from build123d import *

# Parameters (mm, degrees)
F1_DEPTH = 3.75
F2_R     = 1.25
F3_DEPTH = 30


with BuildPart() as f1:
    # F0 (on Front) → F1 (new body)
    with BuildSketch(Plane.XZ):
        Polygon((6.409004, 25.153901), (-3.681577, 25.153901), (-7.50148, 17.153901), (-3.681577, 9.153901), (6.409004, 9.153901), (10.228907, 17.153901), align=None)
    extrude(amount=F1_DEPTH)

    # F2 (on face) → F3 (join)
    with BuildSketch(Plane.XZ.offset(3.75)):
        with Locations((1.363714, 17.153901)):
            Circle(F2_R)
    extrude(amount=F3_DEPTH)


solid = f1.part
Geometry: final body of the model. Coordinates: model frame, mm. A direction names the side the tool comes from. Give positions to 0.01 mm unless a question says otherwise; leave off trailing zeros. Order: outer loops, then holes, each group sorted by start corner. A loop starts at its lowest first (then second) coordinate and runs counter-clockwise, first axis right, second up. Notation, with made-up numbers: (34, 36) - (61, 36) arc R19 ccw to (61, 42) - close; hole circle Ø8 at (-22.5, 54). An arc over 180 degrees is marked (long way). Use CSV: the item, a comma, the result in double quotes.
1. Section query B-B (y = -17). Output: boundary loops of the cut face in (x, z), plus the area to 3 significant figures.
Answers below:
outline,"circle Ø2.5 at (1.36, 17.15)"
area,"4.91 mm2"
2. Contact query for flat-ended pins moving along their axis: pin 1 (3 mm diameter, centred on x = 1.5, y = -14.5, fed in from +Z); pin 2 (1.5 mm diameter, centred on y = -8, z = 20.5, fed in from +X); pin 3 (3 mm diameter, centred on y = -7.5, z = 16.5, fed in from -X). Output: stop coordinate, or through.
Answers below:
pin 1,"z = 18.4"
pin 2,"through"
pin 3,"x = 0.11"
3. Section query A-A (z = 17.75). Output: boundary loops of the cut face in (x, y) (3 decimals), plus the area to 3 significant figures.
Answers below:
outline,"(-7.217, -3.75) - (0.265, -3.75) - (0.265, -33.75) - (2.462, -33.75) - (2.462, -3.75) - (9.944, -3.75) - (9.944, 0) - (-7.217, 0) - close"
area,"130 mm2"
4. Section query D-D (z = 15.25). Output: boundary loops of the cut face in (x, y).
Answers below:
outline,"(-6.59, -3.75) - (9.32, -3.75) - (9.32, 0) - (-6.59, 0) - close"
5. Material intervals for line 1 along Y through (x, z) = (4.5, 11.25); line 2 along X through (y, z) = (-2, 14.25); line 3 along X through (y, z) = (-10, 16.75), sorted ascending. Write a range as from..to.
Answers below:
line 1,"-3.75..0"
line 2,"-6.11..8.84"
line 3,"0.18..2.55"
6. Access query for faces 1 (the face through (1, -2, 25.154)), 2 (the face through (1.201, -18.54, 18.393)). Directions: +Z, -Z, +X, -X, +Y, -Y. A direction counts if a zero-diameter tool reaches every point of the face in a straight line with its end or side. Return the directions, or none.
Answers below:
face 1,"+Z, +X, -X, +Y, -Y"
face 2,"-Y"
7. Section query C-C (x = -0.5). Output: boundary loops of the cut face in (y, z).
Answers below:
outline,"(-3.75, 9.15) - (0, 9.15) - (0, 25.15) - (-3.75, 25.15) - close"
